from build123d import *

# Parameters (mm, degrees)
SKETCH_W     = 90
SKETCH_H     = 122
PAD_DEPTH    = 15
POCKET_DEPTH = 2
SKETCH002_R  = 0.4
PAD001_DEPTH = 10.5


with BuildPart() as part:
    # Sketch → Pad (new body)
    with BuildSketch(Plane.XZ):
        with Locations((45, 61)):
            Rectangle(SKETCH_W, SKETCH_H)
    extrude(amount=PAD_DEPTH)

    # Sketch001 (on Face5 of Pad) → Pocket (cut)
    with BuildSketch(Plane(origin=(0, 0, 0), x_dir=(1, 0, 0), z_dir=(0, 1, 0))):
        Polygon((88, -122), (88, -120), (90, -120), (90, -2), (88, -2), (88, 0), (2, 0), (2, -2), (0, -2), (0, -120), (2, -120), (2, -122), align=None)
    extrude(amount=-POCKET_DEPTH, mode=Mode.SUBTRACT)

    # Sketch002 (on Face4 of Pocket) → Pad001 (join)
    with BuildSketch(Plane(origin=(0, -2, 0), x_dir=(1, 0, 0), z_dir=(0, 1, 0))):
        with Locations((34.84, -7.5)):
            Circle(SKETCH002_R)
        with Locations((39.92, -7.5)):
            Circle(SKETCH002_R)
        with Locations((45, -7.5)):
            Circle(SKETCH002_R)
        with Locations((50.08, -7.5)):
            Circle(SKETCH002_R)
        with Locations((55.16, -7.5)):
            Circle(SKETCH002_R)
        with Locations((34.84, -114.5)):
            Circle(SKETCH002_R)
        with Locations((39.92, -114.5)):
            Circle(SKETCH002_R)
        with Locations((45, -114.5)):
            Circle(SKETCH002_R)
        with Locations((50.08, -114.5)):
            Circle(SKETCH002_R)
        with Locations((55.16, -114.5)):
            Circle(SKETCH002_R)
    extrude(amount=PAD001_DEPTH)


solid = part.part
Model file for the job. Use its own axes, mm. Give positions to 0.01 mm unless a question says otherwise; leave off trailing zeros. Order: outer loops, then holes, each group sorted by start corner. A loop starts at its lowest first (then second) coordinate and runs counter-clockwise, first axis right, second up. Notation, with made-up numbers: M 21,-33.75 L 64,-33.75 A17 ccw 64,-25.75 Z; hole C 81.5,-4.5 d10. An arc over 180 degrees is marked long. Put each result on its own line as item: value. Start each with the question number.
(1) Pin check, flat tips, straight feed: pin 1 Ø0.6 at (x, z) = (0.5, 1) entering from +Y; pin 2 Ø1.5 at (x, y) = (61, -4.5) entering from -Z; pin 3 Ø1 at (x, z) = (23.5, 46.5) entering from +Y. Stop position of each tip, or through.
(2) Band-saw the part on B-B on x = 72. Give the cut face in (y, z), then the cut area to 3 significant figures.
(3) Band-saw the part on C-C on z = 70.5. Give the cut face in (x, y), then the cut area to 3 significant figures.
(4) Drill centre line: L1, parallel to Y at x = 29.5, z = 20. Where is it in solid material? Low to high. Write a range as [from, to].
(5) Band-saw the part on A-A on y = 1.5. Count the separate pieces of the cut face and the enclosed holes in it, then the cut area to 3 significant figures.
Results below:
1. pin 1: stops at y = 0
1. pin 2: stops at z = 0
1. pin 3: stops at y = -2
2. outline: M -15,0 L -2,0 L -2,122 L -15,122 Z
2. area: 1,590 mm2
3. outline: M 0,-15 L 90,-15 L 90,-2 L 0,-2 Z
3. area: 1,170 mm2
4. L1: y = [-15, -2]
5. separate pieces: 10
5. enclosed holes: 0
5. area: 5.03 mm2
